Could you check a few things on this model? Use its own coordinates, in mm. Round coordinates to 2 decimals unless told otherwise and drop trailing zeros. Loops run counter-clockwise (first coordinate to the right, second up) from the corner with the lowest first, then second, coordinate; pieces in that order, holes last. Notation, with made-up numbers: (9, 23) - (65, 23) arc R12 cw to (65, 27) - close; hole circle Ø8 at (-40, 62). An arc over 180 degrees is marked (long way). Answer as CSV lines item,"result". Start each with the question number.
1) Suppose I cut it at B-B, the plane y = 4.5. Write out the boundary of the cut face in (x, z), then the cut area to 3 significant figures.
2) Suppose I cut it at C-C, the plane x = 207.5. Write out the boundary of the cut face in (y, z), then the cut area to 3 significant figures.
3) I'm going to push flat-ended pins straight in: pin 1 Ø7 at (x, z) = (207.5, -15) entering from -Y; pin 2 Ø1.5 at (x, z) = (49, -22) entering from -Y. Where does each tip first touch, or does it pass through?
4) Suppose I cut it at D-D, the plane x = 167.5. Write out the boundary of the cut face in (y, z), then the cut area to 3 significant figures.
5) Suppose I cut it at A-A, the plane x = 142.5. Write out the boundary of the cut face in (y, z), then the cut area to 3 significant figures.
6) Please list where these lines run through material, in increasing order: line 1 along Z through (x, y) = (62.5, 8.6); line 2 along X through (y, z) = (8.4, -15); line 3 along X through (y, z) = (1.5, -22.5).
Autodesk Inventor part; units mm, degrees
ref_plane "YZ Plane" through (0, 0, 0) normal (1, 0, 0) x (0, 1, 0)
ref_plane "XZ Plane" through (0, 0, 0) normal (0, 1, 0) x (-1, 0, 0)
ref_plane "XY Plane" through (0, 0, 0) normal (0, 0, 1) x (1, 0, 0)
sketch "Sketch1" plane through (0, 0, 0) normal (1, 0, 0) x (0, 1, 0)
  point P0 (0, 0)
sketch "Sketch2" plane through (0, 0, 0) normal (1, 0, 0) x (0, 1, 0)
  point P0 (0, 0)
sketch "Sketch3" plane through (0, 0, 0) normal (1, 0, 0) x (0, 1, 0)
  line L0 (0, 0) -> (10, 0)
  line L1 (10, 0) -> (10, -30)
  line L2 (10, -30) -> (0, -30)
  line L3 (0, -30) -> (0, 0)
  line L4 (9, -29) -> (1, -29)
  line L5 (1, -29) -> (1, -1)
  line L6 (1, -1) -> (9, -1)
  line L7 (9, -1) -> (9, -29)
  dimension "d0" = 10
  dimension "d1" = 30
  dimension "d2" = 8
  dimension "d3" = 28
extrude "Extrusion1" add sketch "Sketch3" along normal blind 200 contours L0 L1 L2 L3 | L4 L5 L6 L7
sketch "Sketch4" plane through (200, 0, 0) normal (1, 0, 0) x (0, 0, -1)
  line L0 (29, 9) -> (1, 9)
  line L1 (1, 9) -> (1, 1)
  line L2 (1, 1) -> (29, 1)
  line L3 (29, 1) -> (29, 9)
  point P0 (0, 0)
  dimension "d6" = 28
  dimension "d7" = 8
extrude "Extrusion2" cut sketch "Sketch4" against normal blind 303.2375
sketch "Sketch5" plane through (0, 10, 0) normal (0, 1, 0) x (1, 0, 0)
  point P0 (0, 0)
sketch "Sketch6" plane through (200, 0, 0) normal (1, 0, 0) x (0, 0, -1)
  point P0 (0, 0)
sketch "Sketch7" plane through (200, 0, 0) normal (1, 0, 0) x (0, 0, -1)
  line L0 (0, 0) -> (30, 0)
  line L1 (30, 10) -> (0, 10)
  line L2 (30, 0) -> (0, 0)
  line L3 (0, 0) -> (0, 10)
  line L4 (0, 10) -> (30, 10)
  line L5 (30, 10) -> (30, 0)
extrude "Extrusion3" add sketch "Sketch7" along normal blind 20
sketch "Sketch8" plane through (0, 0, 0) normal (-1, 0, 0) x (0, 0, 1)
  line L0 (-29, 9) -> (-1, 9)
  line L1 (-1, 9) -> (-1, 1)
  line L2 (-1, 1) -> (-29, 1)
  line L3 (-29, 1) -> (-29, 9)
  point P0 (0, 0)
sketch "Sketch9" plane through (220, 0, 0) normal (1, 0, 0) x (0, 0, -1)
  line L0 (1, 1) -> (29, 1)
  line L1 (29, 1) -> (29, 9)
  line L2 (29, 9) -> (1, 9)
  line L3 (1, 9) -> (1, 1)
  point P0 (0, 0)
extrude "Extrusion4" cut sketch "Sketch9" against normal blind 750.25
sketch "Sketch10" plane through (0, 10, 0) normal (0, 1, 0) x (1, 0, 0)
  circle A0 centre (22.5, 15) radius 4
  circle A1 centre (46.5, 15) radius 4
  point P0 (0, 0)
  dimension "d14" = 8
  dimension "d15" = 8
extrude "Extrusion5" cut sketch "Sketch10" against normal blind 63.025
sketch "Sketch11" plane through (0, 10, 0) normal (0, 1, 0) x (1, 0, 0)
  circle A0 centre (173.5, 15) radius 4
  circle A1 centre (197.5, 15) radius 4
  point P0 (0, 0)
  dimension "d18" = 8
  dimension "d19" = 8
extrude "Extrusion6" cut sketch "Sketch11" against normal blind 120.175
sketch "Sketch12" plane through (0, 10, 0) normal (0, 1, 0) x (1, 0, 0)
  line L0 (0, 30) -> (220, 30)
  line L1 (0, 0) -> (220, 0)
  line L2 (0, 30) -> (10, 30)
  line L3 (10, 30) -> (10, 0)
  line L4 (10, 0) -> (0, 0)
  line L5 (0, 0) -> (0, 30)
  dimension "d22" = 10
extrude "Extrusion7" cut sketch "Sketch12" against normal blind 98.9
sketch "Sketch13" plane through (220, 10, 0) normal (0, 1, 0) x (1, 0, 0)
  line L0 (-210, 30) -> (0, 30)
  line L1 (0, 0) -> (-10, 0)
  line L2 (-10, 0) -> (-10, 30)
  line L3 (-10, 30) -> (0, 30)
  line L4 (0, 30) -> (0, 0)
  point P0 (-220, 0)
  dimension "d25" = 10
extrude "Extrusion8" cut sketch "Sketch13" against normal blind 67.7875
sketch "Sketch14" plane through (10, 10, 0) normal (0, 1, 0) x (1, 0, 0)
  circle A0 centre (52.5, 7.5) radius 2.5
  circle A1 centre (52.5, 22.5) radius 2.5
  point P0 (-10, 0)
  dimension "d28" = 5
  dimension "d29" = 5
sketch "Sketch15" plane through (10, 10, 0) normal (0, 1, 0) x (1, 0, 0)
  circle A0 centre (67.5, 22.5) radius 2.5
  circle A1 centre (67.5, 7.5) radius 2.5
  point P0 (-10, 0)
  dimension "d30" = 5
  dimension "d31" = 5
extrude "Extrusion9" cut sketch "Sketch14" against normal blind 97.95
extrude "Extrusion10" cut sketch "Sketch15" against normal blind 108.425
sketch "Sketch16" plane through (10, 10, 0) normal (0, 1, 0) x (1, 0, 0)
  circle A0 centre (147.5, 22.5) radius 2.5
  circle A1 centre (132.5, 22.5) radius 2.5
  circle A2 centre (132.5, 7.5) radius 2.5
  circle A3 centre (147.5, 7.5) radius 2.5
  point P0 (-10, 0)
  dimension "d36" = 5
  dimension "d37" = 5
  dimension "d38" = 5
  dimension "d39" = 5
extrude "Extrusion11" cut sketch "Sketch16" against normal blind 59.85
sketch "Sketch17" plane through (10, 10, 0) normal (0, 1, 0) x (1, 0, 0)
  circle A0 centre (100, 15) radius 4
  point P0 (-10, 0)
  dimension "d42" = 8
extrude "Extrusion12" cut sketch "Sketch17" against normal blind 53.5
sketch "Sketch20" plane through (10, 10, -30) normal (-1, 0, 0) x (0, 0, 1)
  line L0 (30, -10) -> (0, -10)
  line L1 (30, 0) -> (0, 0)
  line L2 (30, -10) -> (0, -10)
  line L3 (0, -10) -> (0, 0)
  line L4 (0, 0) -> (30, 0)
  line L5 (30, 0) -> (30, -10)
  line L6 (29, -9) -> (1, -9)
  line L7 (29, -1) -> (1, -1)
  line L8 (29, -9) -> (1, -9)
  line L9 (1, -9) -> (1, -1)
  line L10 (1, -1) -> (29, -1)
  line L11 (29, -1) -> (29, -9)
extrude "Extrusion13" add sketch "Sketch20" along normal blind 10 contours L0 L3 L1 L5 | L6 L9 L7 L11
extrude "Extrusion14" cut sketch "Sketch8" against normal blind 34.45
sketch "Sketch21" plane through (210, 10, 0) normal (1, 0, 0) x (0, 0, -1)
  line L0 (30, -10) -> (0, -10)
  line L1 (0, 0) -> (30, 0)
  line L2 (30, 0) -> (30, -10)
  line L3 (30, -10) -> (0, -10)
  line L4 (0, -10) -> (0, 0)
  line L5 (29, -1) -> (1, -1)
  line L6 (1, -9) -> (29, -9)
  line L7 (1, -1) -> (29, -1)
  line L8 (29, -1) -> (29, -9)
  line L9 (29, -9) -> (1, -9)
  line L10 (1, -9) -> (1, -1)
extrude "Extrusion15" add sketch "Sketch21" along normal blind 10 contours L0 L4 L1 L2 | L8 L6 L10 L5
sketch "Sketch22" plane through (220, 10, 0) normal (1, 0, 0) x (0, 0, -1)
  point P0 (0, -10)
sketch "Sketch23" plane through (220, 10, 0) normal (1, 0, 0) x (0, 0, -1)
  point P0 (0, -10)
sketch "Sketch24" plane through (0, 10, -30) normal (-1, 0, 0) x (0, 0, 1)
  line L0 (2, -2) -> (28, -2)
  line L1 (28, -2) -> (28, -8)
  line L2 (28, -8) -> (2, -8)
  line L3 (2, -8) -> (2, -2)
  point P0 (30, -10)
  dimension "d51" = 26
  dimension "d52" = 6
extrude "Extrusion16" add sketch "Sketch24" against normal blind 220
sketch "Sketch25" plane through (220, 10, 0) normal (1, 0, 0) x (0, 0, -1)
  line L0 (2, -8) -> (2, -2)
  line L1 (28, -2) -> (28, -8)
  line L2 (2, -8) -> (28, -8)
  line L3 (28, -8) -> (28, -2)
  line L4 (28, -2) -> (2, -2)
  line L5 (2, -2) -> (2, -8)
  point P0 (0, -10)
extrude "Extrusion17" cut sketch "Sketch25" against normal blind 351.5
sketch "Sketch26" plane through (210, 10, 0) normal (-1, 0, 0) x (0, 0, 1)
  point P0 (0, -10)
sketch "Sketch27" plane through (0, 10, -30) normal (-1, 0, 0) x (0, 0, 1)
  line L0 (2, -2) -> (2, -8)
  line L1 (2, -8) -> (28, -8)
  line L2 (2, -2) -> (28, -2)
  line L3 (28, -2) -> (28, -8)
  line L4 (28, -8) -> (2, -8)
  line L5 (2, -8) -> (2, -2)
  line L6 (29, -1) -> (29, -9)
  line L7 (29, -9) -> (0.9924, -9)
  line L8 (0.9924, -9) -> (0.9924, -1)
  line L9 (0.9924, -1) -> (29, -1)
  line L10 (29, -1) -> (29, -9)
  point P0 (30, -10)
extrude "Extrusion18" cut sketch "Sketch27" against normal blind 220
sketch "Sketch28" plane through (220, 10, 0) normal (1, 0, 0) x (0, 0, -1)
  line L0 (2, -8) -> (28, -8)
  line L1 (28, -8) -> (28, -2)
  line L2 (28, -2) -> (2, -2)
  line L3 (2, -2) -> (2, -8)
  line L4 (29.0076, -1) -> (1, -1)
  line L5 (1, -9) -> (29.0076, -9)
  line L6 (1, -1) -> (29.0076, -1)
  line L7 (29.0076, -1) -> (29.0076, -9)
  line L8 (29.0076, -9) -> (1, -9)
  line L9 (1, -9) -> (1, -1)
  point P0 (0, -10)
  dimension "d59" = 26
  dimension "d60" = 6
extrude "Extrusion19" add sketch "Sketch28" against normal blind 220
sketch "Sketch29" plane through (0, 10, 0) normal (0, 1, 0) x (1, 0, 0)
  circle A0 centre (12.5, 15) radius 4
  point P0 (0, 0)
  dimension "d63" = 8
sketch "Sketch30" plane through (0, 10, 0) normal (0, 1, 0) x (1, 0, 0)
  circle A0 centre (36.5, 15) radius 4
  point P0 (0, 0)
  dimension "d64" = 8
extrude "Extrusion20" cut sketch "Sketch30" against normal blind 143.5375
extrude "Extrusion21" cut sketch "Sketch29" against normal blind 377.1625
sketch "Sketch31" plane through (22.5, 9, -15) normal (0, 1, 0) x (1, 0, 0)
  circle A0 centre (0, 0) radius 4
  circle A1 centre (24, 0) radius 4
  point P0 (-22.5, -15)
extrude "Extrusion22" cut sketch "Sketch31" against normal blind 135.6
sketch "Sketch32" plane through (0, 10, 0) normal (0, 1, 0) x (1, 0, 0)
  circle A0 centre (22.5, 15) radius 4
  circle A1 centre (22.5, 15) radius 4
  circle A2 centre (46.5, 15) radius 4
  circle A3 centre (46.5, 15) radius 4
  point P0 (0, 0)
extrude "Extrusion23" add sketch "Sketch32" against normal blind 2
sketch "Sketch33" plane through (0, 0, -30) normal (0, -1, 0) x (1, 0, 0)
  circle A0 centre (46.5, 14.9969) radius 4
  circle A1 centre (22.5, 14.9969) radius 4
  point P0 (0, 30)
  dimension "d73" = 8
  dimension "d74" = 8
extrude "Extrusion24" add sketch "Sketch33" against normal blind 2
sketch "Sketch36" plane through (0, 10, 0) normal (0, 1, 0) x (1, 0, 0)
  circle A0 centre (207.5, 15) radius 4
  circle A1 centre (183.5, 15) radius 4
  point P0 (0, 0)
  dimension "d77" = 8
  dimension "d78" = 8
extrude "Extrusion25" cut sketch "Sketch36" against normal blind 72.6125
sketch "Sketch37" plane through (0, 10, 0) normal (0, 1, 0) x (1, 0, 0)
  circle A0 centre (197.5, 15) radius 4
  circle A1 centre (197.5, 15) radius 4
  circle A2 centre (173.5, 15) radius 4
  circle A3 centre (173.5, 15) radius 4
  point P0 (0, 0)
extrude "Extrusion26" add sketch "Sketch37" against normal blind 2
sketch "Sketch38" plane through (0, 0, -30) normal (0, -1, 0) x (1, 0, 0)
  circle A0 centre (173.5, 15) radius 4
  circle A1 centre (173.5, 15) radius 4
  circle A2 centre (197.5, 15) radius 4
  circle A3 centre (197.5, 15) radius 4
  point P0 (0, 30)
extrude "Extrusion27" add sketch "Sketch38" against normal blind 2
sketch "Sketch39" plane through (0, 0, -30) normal (0, -1, 0) x (1, 0, 0)
  circle A0 centre (62.5, 22.5) radius 2.5
  circle A1 centre (62.5, 22.5) radius 2.5
  circle A2 centre (77.5, 22.5) radius 2.5
  circle A3 centre (77.5, 22.5) radius 2.5
  circle A4 centre (77.5, 7.5) radius 2.5
  circle A5 centre (77.5, 7.5) radius 2.5
  circle A6 centre (62.5, 7.5) radius 2.5
  circle A7 centre (62.5, 7.5) radius 2.5
  circle A8 centre (142.5, 22.5) radius 2.5
  circle A9 centre (142.5, 22.5) radius 2.5
  circle A10 centre (157.5, 22.5) radius 2.5
  circle A11 centre (157.5, 22.5) radius 2.5
  circle A12 centre (157.5, 7.5) radius 2.5
  circle A13 centre (157.5, 7.5) radius 2.5
  circle A14 centre (142.5, 7.5) radius 2.5
  circle A15 centre (142.5, 7.5) radius 2.5
  circle A16 centre (110, 15) radius 4
  circle A17 centre (110, 15) radius 4
  point P0 (0, 30)
extrude "Extrusion28" cut sketch "Sketch39" against normal blind 68.675
properties part number "short_frame" material "Aluminum 6061"
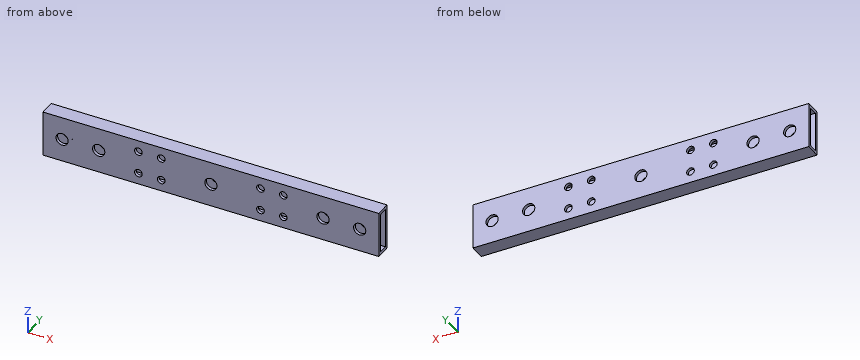
Filled sheet:
1,outline,"(0, -30) - (220, -30) - (220, -28) - (0, -28) - close; (0, -2) - (220, -2) - (220, 0) - (0, 0) - close"
1,area,"880 mm²"
2,outline,"(0, -30) - (10, -30) - (10, -19) - (8, -19) - (8, -28) - (2, -28) - (2, -19) - (0, -19) - close; (0, -11) - (2, -11) - (2, -2) - (8, -2) - (8, -11) - (10, -11) - (10, 0) - (0, 0) - close"
2,area,"112 mm²"
3,pin 1,"through"
3,pin 2,"y = 0"
4,outline,"(0, -30) - (10, -30) - (10, 0) - (0, 0) - close; hole (2, -28) - (8, -28) - (8, -2) - (2, -2) - close"
4,area,"144 mm²"
5,outline,"(0, -30) - (10, -30) - (10, -25) - (8, -25) - (8, -28) - (2, -28) - (2, -25) - (0, -25) - close; (0, -20) - (2, -20) - (2, -10) - (0, -10) - close; (0, -5) - (2, -5) - (2, -2) - (8, -2) - (8, -5) - (10, -5) - (10, 0) - (0, 0) - close; (8, -20) - (10, -20) - (10, -10) - (8, -10) - close"
5,area,"104 mm²"
6,line 1,"-30 to -25, -20 to -10, -5 to 0"
6,line 2,"0 to 8.5, 16.5 to 32.5, 40.5 to 106, 114 to 179.5, 187.5 to 203.5, 211.5 to 220"
6,line 3,"0 to 60, 65 to 75, 80 to 140, 145 to 155, 160 to 220"
